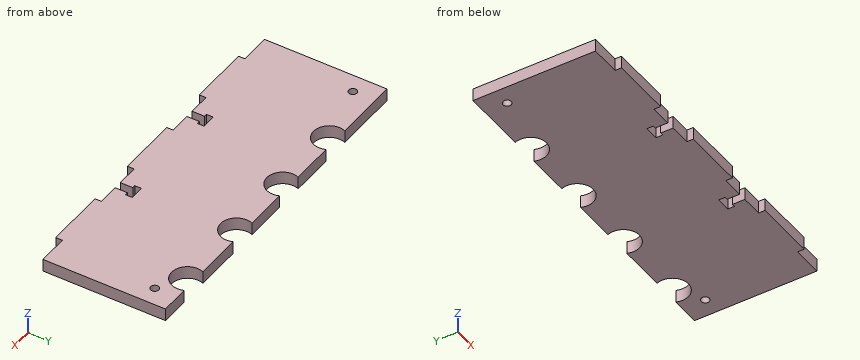
Autodesk Inventor part; units mm, degrees
ref_plane "YZ Plane" through (0, 0, 0) normal (1, 0, 0) x (0, 1, 0)
ref_plane "XZ Plane" through (0, 0, 0) normal (0, 1, 0) x (-1, 0, 0)
ref_plane "XY Plane" through (0, 0, 0) normal (0, 0, 1) x (1, 0, 0)
sketch "Sketch1" plane through (0, 0, 0) normal (0, 0, 1) x (1, 0, 0)
  circle A0 centre (0.15, -0.0866) radius 7.5
  circle A1 centre (35.6226, -0.0866) radius 7.5
  line L0 (-37.4458, 2.8981) -> (-34.0994, 2.8981)
  line L1 (-39.119, 0) -> (-37.4458, 2.8981)
  line L2 (-37.4458, -2.8981) -> (-39.119, 0)
  line L3 (-34.0994, -2.8981) -> (-37.4458, -2.8981)
  line L4 (-32.4262, 0) -> (-34.0994, -2.8981)
  line L5 (-34.0994, 2.8981) -> (-32.4262, 0)
  line L6 (71.3985, 2.8989) -> (74.7449, 2.8989)
  line L7 (69.7253, 0.0008) -> (71.3985, 2.8989)
  line L8 (71.3985, -2.8973) -> (69.7253, 0.0008)
  line L9 (74.7449, -2.8973) -> (71.3985, -2.8973)
  line L10 (76.4181, 0.0008) -> (74.7449, -2.8973)
  line L11 (74.7449, 2.8989) -> (76.4181, 0.0008)
  line L12 (94.8132, 2.8981) -> (94.8132, -57.1019)
  line L13 (-75.1868, -57.1019) -> (-75.1868, 2.8981)
  line L14 (-75.1868, 2.8981) -> (94.8132, 2.8981)
  circle A2 centre (-35.6226, -0.0866) radius 7.5
  circle A3 centre (73.2223, -0.0862) radius 7.5
  circle A4 centre (-35.6226, -0.0866) radius 7.8
  circle A5 centre (0.15, -0.0866) radius 7.8
  circle A6 centre (35.6226, -0.0866) radius 7.8
  circle A7 centre (73.2223, -0.0862) radius 7.8
  circle A8 centre (85.8132, -8.0862) radius 2
  line L15 (73.2223, -0.0862) -> (73.2223, 6.7764) construction
  circle A9 centre (-66.1868, -8.0866) radius 2
  line L16 (95, -57.1019) -> (-75.1868, -57.1019)
  line L17 (-60.1868, -57.1019) -> (-30.1868, -57.1019)
  line L18 (-30.1868, -57.1019) -> (-30.1868, -60.3019)
  line L19 (-30.1868, -60.3019) -> (-60.1868, -60.3019)
  line L20 (-60.1868, -60.3019) -> (-60.1868, -57.1019)
  line L21 (9.9066, -57.1019) -> (9.9066, -41.5844) construction
  line L22 (9.9066, -57.1019) -> (9.9066, -60.3019)
  line L23 (9.9066, -60.3019) -> (-5.0934, -60.3019)
  line L24 (-5.0934, -60.3019) -> (-5.0934, -57.1019)
  line L25 (50, -57.1019) -> (50, -60.3019)
  line L26 (50, -60.3019) -> (80, -60.3019)
  line L27 (80, -60.3019) -> (80, -57.1019)
  line L28 (9.9066, -60.3019) -> (24.9066, -60.3019)
  line L29 (24.9066, -60.3019) -> (24.9066, -57.1019)
  point P0 (0, 0)
  point P1 (80.4289, 2.8981)
  point P2 (66.0158, 2.8981)
  point P3 (42.8289, 2.8981)
  point P4 (28.4162, 2.8981)
  point P5 (7.3564, 2.8981)
  point P6 (-7.0564, 2.8981)
  point P7 (-28.4162, 2.8981)
  point P8 (-42.8289, 2.8981)
  point P9 (94.8132, -57.1019)
  point P10 (-30.1868, -57.1019)
  point P11 (24.9066, -57.1019)
  point P12 (50, -57.1019)
  point P13 (80, -57.1019)
  dimension "d2" = 170
  dimension "d4" = 0.3
  dimension "d5" = 0.3
  dimension "d6" = 0.3
  dimension "d7" = 0.3
  dimension "d17" = 4
  dimension "d19" = 8
  dimension "d24" = 9
  dimension "d42" = 60
  dimension "d43" = 30
  dimension "d44" = 3.2
  dimension "d45" = 15
  dimension "d46" = 75.1868
  dimension "d47" = 94.8132
  dimension "d48" = 9
  dimension "d49" = 8
  dimension "d50" = 4
  dimension "d51" = 3.2
  dimension "d52" = 15
  dimension "d53" = 25.0934
extrude "Extrusion3" add sketch "Sketch1" along normal blind 0.1 and the other way blind 6.1 contours L14 A6 A7 L12 L16 L13 A4 A5 | L16 L18 L19 L20 | L27 L26 L25 L16 | L16 L22 L23 L24 | L16 L29 L28 L22
sketch "Sketch2" plane through (0, 0, 0.1) normal (0, 0, 1) x (1, 0, 0)
  line L0 (-5.0934, -60.3019) -> (24.9066, -60.3019)
  line L1 (24.9066, -60.3019) -> (-5.0934, -60.3019)
  line L2 (9.9066, -60.3019) -> (9.9066, -41.2301) construction
  line L3 (-30.1868, -57.1019) -> (-5.0934, -57.1019)
  line L4 (-17.6401, -57.1019) -> (-17.6401, -48.823) construction
  line L5 (-19.6401, -57.1019) -> (-15.6401, -57.1019)
  line L6 (-15.6401, -57.1019) -> (-15.6401, -51.0019)
  line L7 (-19.6401, -51.0019) -> (-19.6401, -57.1019)
  line L8 (-17.6401, -51.0019) -> (-14.1401, -51.0019)
  line L9 (-14.1401, -51.0019) -> (-14.1401, -47.8019)
  line L10 (-19.6401, -51.0019) -> (-15.6401, -51.0019)
  line L11 (-17.6401, -51.0019) -> (-21.1401, -51.0019)
  line L12 (-21.1401, -51.0019) -> (-21.1401, -47.8019)
  line L13 (-21.1401, -47.8019) -> (-14.1401, -47.8019)
  line L14 (37.4533, -57.1019) -> (37.4533, -48.823) construction
  line L15 (39.4533, -57.1019) -> (35.4533, -57.1019)
  line L16 (35.4533, -57.1019) -> (35.4533, -51.0019)
  line L17 (39.4533, -51.0019) -> (39.4533, -57.1019)
  line L18 (37.4533, -51.0019) -> (33.9533, -51.0019)
  line L19 (33.9533, -51.0019) -> (33.9533, -47.8019)
  line L20 (39.4533, -51.0019) -> (35.4533, -51.0019)
  line L21 (37.4533, -51.0019) -> (40.9533, -51.0019)
  line L22 (40.9533, -51.0019) -> (40.9533, -47.8019)
  line L23 (40.9533, -47.8019) -> (33.9533, -47.8019)
  point P0 (0, 0)
  dimension "d64" = 2
  dimension "d65" = 3.5
  dimension "d66" = 3.2
  dimension "d67" = 4
  dimension "d68" = 6.1
  dimension "d69" = 7
extrude "Extrusion4" cut sketch "Sketch2" against normal blind 7
properties part number "Carcasa_CajaR_Lateral1"
Model file for the job. Use its own axes, mm. Coordinates: 2 decimals unless noted, no trailing zeros. Write each loop counter-clockwise with the first axis right and the second up, starting at its lowest first coordinate (ties: lowest second). Pieces come first, ordered by that corner, then holes. Notation, with made-up numbers: (21, 66.25) - (27, 66.25) arc R11 cw to (27, 83.25) - close; hole circle Ø6 at (-31.75, -28). An arc over 180 degrees is marked (long way). Use a Markdown table: item, result. Add a question column.
Item 1: Band-saw the part on A-A, the plane y = -2. Write the cut outline in (x, z).
Item 2: Band-saw the part on D-D, the plane x = 37. Write the cut outline in (y, z), and give its area (3 significant figures).
Item 3: Band-saw the part on B-B, the plane x = 0.15. Write the cut outline in (y, z).
Item 4: Band-saw the part on C-C, the plane z = -3. Give the number of separate pieces and of enclosed holes in the cut face, and give its area (3 significant figures).
Item 5: Drill centre lines: line 1 along X through (y, z) = (-57.5, -3.25); line 2 along X through (y, z) = (-53, -1); line 3 along Y through (x, z) = (35, -0.25). Where is each one in solid material? Low to high.
Item 6: Drop flat-ended pins along their axis: pin 1 (3 mm diameter, centred on x = -66.5, z = -4.5, fed in from -Y); pin 2 (1.2 mm diameter, centred on x = 40.5, z = -4, fed in from +Y); pin 3 (1 mm diameter, centred on y = -58, z = -3.5, fed in from -X). Give the stop position or say it passes through.
A:
| question | item | result |
|---|---|---|
| 1 | outline | (-75.19, -6.1) - (-43.18, -6.1) - (-43.18, 0.1) - (-75.19, 0.1) - close; (-28.06, -6.1) - (-7.41, -6.1) - (-7.41, 0.1) - (-28.06, 0.1) - close; (7.71, -6.1) - (28.06, -6.1) - (28.06, 0.1) - (7.71, 0.1) - close; (43.18, -6.1) - (65.66, -6.1) - (65.66, 0.1) - (43.18, 0.1) - close; (80.78, -6.1) - (94.81, -6.1) - (94.81, 0.1) - (80.78, 0.1) - close |
| 2 | outline | (-47.8, -6.1) - (-7.76, -6.1) - (-7.76, 0.1) - (-47.8, 0.1) - close |
| 2 | area | 248 mm² |
| 3 | outline | (-60.3, -6.1) - (-7.89, -6.1) - (-7.89, 0.1) - (-60.3, 0.1) - close |
| 4 | separate pieces | 1 |
| 4 | enclosed holes | 2 |
| 4 | area | 9,810 mm² |
| 5 | line 1 | x = -60.19 to -30.19, -5.09 to 24.91, 50 to 80 |
| 5 | line 2 | x = -75.19 to -19.64, -15.64 to 35.45, 39.45 to 94.81 |
| 5 | line 3 | y = -57.1 to -51, -47.8 to -7.86 |
| 6 | pin 1 | stops at y = -57.1 |
| 6 | pin 2 | stops at y = -5.64 |
| 6 | pin 3 | stops at x = -60.19 |
